```python
from build123d import *

# Parameters (mm, degrees)
F0_R     = 4.1575260002
F1_DEPTH = 3.81
F2_W     = 4.9914508127
F2_H     = 15.2679625899
F2_W_2   = 15.267963754
F2_H_2   = 4.9914494157
F3_DEPTH = 0.508


# Not quite as in the source:
# - a fillet or chamfer that OpenCascade refuses, or shapes differently, is made with other operations: its cross-section is extruded or revolved along the edge and cut away or added


with BuildPart() as f1:
    # F0 (on Front) → F1 (new body)
    with BuildSketch(Plane.XZ):
        Circle(F0_R)
    extrude(amount=F1_DEPTH)

    # F2 (on Front) → F3 (join)
    with BuildSketch(Plane.XZ):
        with Locations((0, 10.1297060028)):
            Rectangle(F2_W, F2_H)
        with Locations((-10.1297072833, 0)):
            Rectangle(F2_W_2, F2_H_2)
        Rectangle(F2_W, F2_H_2)
        with Locations((0, -10.1297060028)):
            Rectangle(F2_W, F2_H)
        with Locations((10.1297072833, 0)):
            Rectangle(F2_W_2, F2_H_2)
    extrude(amount=F3_DEPTH)

    # F4: fillet of radius 3.81 on 1 edges, made by hand


with BuildPart() as f4_tool2:
    # F4_s3 → F4_t4 (revolve)
    with BuildSketch(Plane.XY):
        with BuildLine():
            ThreePointArc((4.1575260002, 0), (3.0416028366, -2.6940768363), (0.3475260002, -3.81))
            Line((0.3475260002, -3.81), (4.1575260002, -3.81))
            Line((4.1575260002, -3.81), (4.1575260002, 0))
        make_face()
    revolve(axis=Axis((0, -3.81, 0), (0, -1, 0)))

    split(bisect_by=Plane.XZ.offset(0.508), keep=Keep.TOP)


with BuildPart() as f1_1:
    add(f1.part)

    # F4_t1: cut F4_tool2
    add(f4_tool2.part, mode=Mode.SUBTRACT)


with BuildPart() as f4_tool7:
    # F4_s8 → F4_t9 (revolve)
    with BuildSketch(Plane.XY):
        with BuildLine():
            ThreePointArc((4.1575260002, 0), (3.0416028366, -2.6940768363), (0.3475260002, -3.81))
            Line((0.3475260002, -3.81), (4.1575260002, -3.81))
            Line((4.1575260002, -3.81), (4.1575260002, 0))
        make_face()
    revolve(axis=Axis((0, -3.81, 0), (0, -1, 0)))

    split(bisect_by=Plane.XY.offset(2.4957247078), keep=Keep.TOP)

    split(bisect_by=Plane.YZ.offset(2.4957254063), keep=Keep.TOP)


with BuildPart() as f1_2:
    add(f1_1.part)

    # F4_t6: cut F4_tool7
    add(f4_tool7.part, mode=Mode.SUBTRACT)


with BuildPart() as f4_tool13:
    # F4_s14 → F4_t15 (revolve)
    with BuildSketch(Plane.XY):
        with BuildLine():
            ThreePointArc((4.1575260002, 0), (3.0416028366, -2.6940768363), (0.3475260002, -3.81))
            Line((0.3475260002, -3.81), (4.1575260002, -3.81))
            Line((4.1575260002, -3.81), (4.1575260002, 0))
        make_face()
    revolve(axis=Axis((0, -3.81, 0), (0, -1, 0)))

    split(bisect_by=Plane.XY.offset(-2.4957247078), keep=Keep.BOTTOM)

    split(bisect_by=Plane.YZ.offset(2.4957254063), keep=Keep.TOP)


with BuildPart() as f1_3:
    add(f1_2.part)

    # F4_t12: cut F4_tool13
    add(f4_tool13.part, mode=Mode.SUBTRACT)


with BuildPart() as f4_tool19:
    # F4_s20 → F4_t21 (revolve)
    with BuildSketch(Plane.XY):
        with BuildLine():
            ThreePointArc((4.1575260002, 0), (3.0416028366, -2.6940768363), (0.3475260002, -3.81))
            Line((0.3475260002, -3.81), (4.1575260002, -3.81))
            Line((4.1575260002, -3.81), (4.1575260002, 0))
        make_face()
    revolve(axis=Axis((0, -3.81, 0), (0, -1, 0)))

    split(bisect_by=Plane.XY.offset(2.4957247078), keep=Keep.TOP)

    split(bisect_by=Plane.YZ.offset(-2.4957254063), keep=Keep.BOTTOM)


with BuildPart() as f1_4:
    add(f1_3.part)

    # F4_t18: cut F4_tool19
    add(f4_tool19.part, mode=Mode.SUBTRACT)


with BuildPart() as f4_tool25:
    # F4_s26 → F4_t27 (revolve)
    with BuildSketch(Plane.XY):
        with BuildLine():
            ThreePointArc((4.1575260002, 0), (3.0416028366, -2.6940768363), (0.3475260002, -3.81))
            Line((0.3475260002, -3.81), (4.1575260002, -3.81))
            Line((4.1575260002, -3.81), (4.1575260002, 0))
        make_face()
    revolve(axis=Axis((0, -3.81, 0), (0, -1, 0)))

    split(bisect_by=Plane.XY.offset(-2.4957247078), keep=Keep.BOTTOM)

    split(bisect_by=Plane.YZ.offset(-2.4957254063), keep=Keep.BOTTOM)


with BuildPart() as f1_5:
    add(f1_4.part)

    # F4_t24: cut F4_tool25
    add(f4_tool25.part, mode=Mode.SUBTRACT)


solid = f1_5.part
```
Verification items for the finished model (mm, model axes). Round coordinates to 2 decimals unless told otherwise and drop trailing zeros. Order: outer loops, then holes, each group sorted by start corner. A loop starts at its lowest first (then second) coordinate and runs counter-clockwise, first axis right, second up. Notation, with made-up numbers: (37.5, -35.5) - (94.5, -35.5) arc R28 cw to (94.5, -9.5) - close; hole circle Ø10 at (42.25, 1.25). An arc over 180 degrees is marked (long way). Use CSV: the item, a comma, the result in double quotes.
(1) Section check A-A on z = -10.5. Record the boundary of the cut face in (x, y).
Entries:
outline,"(-2.5, -0.51) - (2.5, -0.51) - (2.5, 0) - (-2.5, 0) - close"
(2) Section check B-B on x = -8. Record the boundary of the cut face in (y, z), and give its area (3 significant figures).
Entries:
outline,"(-0.51, -2.5) - (0, -2.5) - (0, 2.5) - (-0.51, 2.5) - close"
area,"2.54 mm^2"
(3) Gauge pin test, flat ends, axial feed: pin 1 Ø2.5 at (x, z) = (10, 1) entering from -Y; pin 2 Ø0.6 at (y, z) = (0, -7) entering from -X; pin 3 Ø8 at (x, z) = (1, -7) entering from -Y. Record the tip position at first contact, or that the pin passes through.
Entries:
pin 1,"y = -0.51"
pin 2,"x = -2.5"
pin 3,"y = -2.66"
(4) Thickness scan on probe 1 along Y at (x, z) = (10, 1.5); probe 2 along X at (y, z) = (-0.35, 14.5). Record the ranges inside material, lowest first. Write a range as from..to.
Entries:
probe 1,"-0.51..0"
probe 2,"-2.5..2.5"
